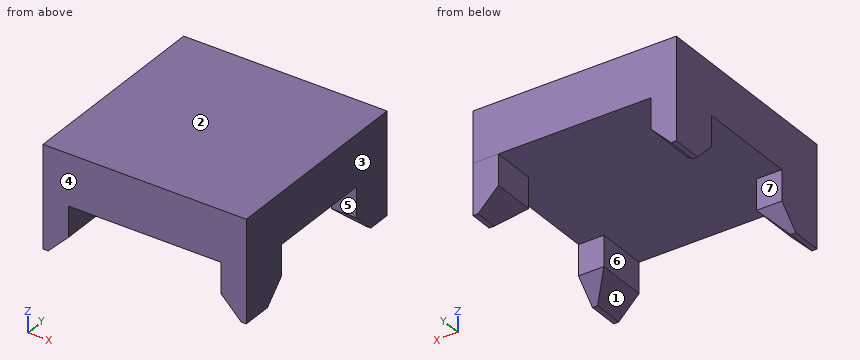
from build123d import *

# Parameters (mm, degrees)
F0_W     = 50.8
F0_H     = 50.8
F1_DEPTH = 12.7
F2_W     = 6.35
F2_H     = 12.7
F2_H_2   = 10.934927
F3_DEPTH = 12.7
F4_SIZE  = 5.08


with BuildPart() as f1:
    # F0 (on Top) → F1 (new body)
    with BuildSketch(Plane.XY):
        with Locations((0.767379, -0.027555)):
            Rectangle(F0_W, F0_H)
    extrude(amount=-F1_DEPTH)

    # F2 (on face) → F3 (join)
    with BuildSketch(Plane(origin=(0, 0, -12.7), x_dir=(1, 0, 0), z_dir=(0, 0, -1))):
        with Locations((-21.457621, 19.077555)):
            Rectangle(F2_W, F2_H)
        with Locations((22.992379, 19.077555)):
            Rectangle(F2_W, F2_H)
        with Locations((-21.457621, -19.022445)):
            Rectangle(F2_W, F2_H)
        with Locations((22.992379, -19.904981)):
            Rectangle(F2_W, F2_H_2)
    extrude(amount=F3_DEPTH)

    # F4
    f4_edges = [f1.edges().sort_by_distance(p)[0] for p in [
        (-21.457621, -12.727555, -25.4),
        (-18.282621, -19.077555, -25.4),
        (19.817379, -19.077555, -25.4),
        (22.992379, -12.727555, -25.4),
        (-18.282621, 19.022445, -25.4),
        (-21.457621, 12.672445, -25.4),
        (22.992379, 14.437518, -25.4),
        (19.817379, 19.904981, -25.4),
    ]]
    chamfer(f4_edges, length=F4_SIZE)


solid = f1.part
The model under review builds one solid part; all positions refer to its coordinate system, in mm. Face numbers are marked on the shaded views. A direction names the side the tool comes from. Round coordinates to 2 decimals unless told otherwise and drop trailing zeros. Order: outer loops, then holes, each group sorted by start corner. A loop starts at its lowest first (then second) coordinate and runs counter-clockwise, first axis right, second up. Notation, with made-up numbers: (32, 63) -> (87, 63) arc R14 ccw to (87, 70) -> close; hole circle Ø1 at (66, 34). An arc over 180 degrees is marked (long way). Return JSON: item names as keys, results as strings.
1. For L1, parallel to Z at x = -22, y = 4.5; L2, parallel to Y at x = -19, z = -15.5; L3, parallel to Y at x = 22, z = -13.75, list the stretches that pass through material, from the lowest coordinate up. Write a range as [from, to].
Answer block:
{"L1": "z = [-12.7, 0]", "L2": "y = [-25.43, -12.73], [12.67, 25.37]", "L3": "y = [-25.43, -12.73], [14.44, 25.37]"}
2. The part is to be moulded in two halves that separate along X. For the marked faces 1, 2 and 3, say which applies: +X half, -X half, draft (parallel to the pull), parting line (faces both ways), or undercut.
Answer block:
{"face 1": "undercut", "face 2": "draft", "face 3": "+X half"}
3. Take a section at B-B (y = -14.5). Write out the cut boundary in (x, z), then the cut area to 3 significant figures.
Answer block:
{"outline": "(-24.63, -22.09) -> (-20.06, -22.09) -> (-18.28, -20.32) -> (-18.28, -12.7) -> (19.82, -12.7) -> (19.82, -20.32) -> (21.59, -22.09) -> (26.17, -22.09) -> (26.17, 0) -> (-24.63, 0) -> close", "area": "761 mm²"}
4. Take a section at A-A (z = -13.5). Write out the cut boundary in (x, y), then the cut area to 3 significant figures.
Answer block:
{"outline": "(-24.63, -25.43) -> (-18.28, -25.43) -> (-18.28, -12.73) -> (-24.63, -12.73) -> close; (-24.63, 12.67) -> (-18.28, 12.67) -> (-18.28, 25.37) -> (-24.63, 25.37) -> close; (19.82, -25.43) -> (26.17, -25.43) -> (26.17, -12.73) -> (19.82, -12.73) -> close; (19.82, 14.44) -> (26.17, 14.44) -> (26.17, 25.37) -> (19.82, 25.37) -> close", "area": "311 mm²"}
5. Take a section at D-D (y = 16.5). Write out the cut boundary in (x, z).
Answer block:
{"outline": "(-24.63, -24.15) -> (-22.11, -24.15) -> (-18.28, -20.32) -> (-18.28, -12.7) -> (19.82, -12.7) -> (19.82, -20.32) -> (21.88, -22.38) -> (26.17, -22.38) -> (26.17, 0) -> (-24.63, 0) -> close"}
6. For the marked faces 4, 5, 6 and 7, list the 3-axis set-ups (+Z, -Z, +X, -X, +Y, -Y) from which the entire face can be reached by the end or side of a thin tool; tool diameter is ignored.
Answer block:
{"face 4": "+Z, -Z, +X, -X, -Y", "face 5": "-Z, +X", "face 6": "-Z, +Y, -Y", "face 7": "-Z, +X, -X"}
7. Take a section at C-C (x = -6). Write out the cut boundary in (y, z), then the cut area to 3 significant figures.
Answer block:
{"outline": "(-25.43, -12.7) -> (25.37, -12.7) -> (25.37, 0) -> (-25.43, 0) -> close", "area": "645 mm²"}
8. Insertion check: P1, Ø10, axis at y = 9.5, z = -20, coming from the +X side; P2, Ø5, axis at x = 19.5, y = 2.5, coming from the -Z side. Each pin has a flat end and moves straight along its axis. Give the tip position at first contact, or say it passes through.
Answer block:
{"P1": "stops at x = 26.17", "P2": "stops at z = -12.7"}
